Work out the finished part from the listing and answer in its coordinate system (mm). Round coordinates to 2 decimals unless told otherwise and drop trailing zeros. Write each loop counter-clockwise with the first axis right and the second up, starting at its lowest first coordinate (ties: lowest second). Pieces come first, ordered by that corner, then holes. Notation, with made-up numbers: M -40,55 L -35,55 A22 ccw -35,92 Z; hole C 73.25,-22.75 d11. An arc over 180 degrees is marked long. Answer in a Markdown table with one row per item.
```python
from build123d import *

# Parameters (mm, degrees)
SKETCH_1_R          = 10
EXTRUDE_1_DEPTH     = 3
SKETCH_3_R          = 0.75
CUT_EXTRUDE_2_DEPTH = 15.456832295
SKETCH_4_R          = 1.8
CUT_EXTRUDE_3_DEPTH = 15.456832295
CUT_EXTRUDE_6_REACH = 16.457


with BuildPart() as part:
    # 草图1 → 凸台-拉伸1 (new body)
    with BuildSketch(Plane(origin=(0, 0, 0), x_dir=(1, 0, 0), z_dir=(0, 1, 0))):
        with Locations(Location((0, 0, 0), (0, 0, 270))):
            Circle(SKETCH_1_R)
    extrude(amount=EXTRUDE_1_DEPTH)

    # 草图3 → 切除-拉伸2 (cut, through all)
    with BuildSketch(Plane(origin=(0, 3, 0), x_dir=(1, 0, 0), z_dir=(0, 1, 0))):
        with Locations(Location((0, 8, 0), (0, 0, 270))):
            Circle(SKETCH_3_R)
        with Locations(Location((2.736161147, 7.517540966, 0), (0, 0, 270))):
            Circle(SKETCH_3_R)
        with Locations(Location((5.142300877, 6.128355545, 0), (0, 0, 270))):
            Circle(SKETCH_3_R)
        with Locations(Location((6.92820323, 4, 0), (0, 0, 270))):
            Circle(SKETCH_3_R)
        with Locations(Location((7.878462024, 1.389185421, 0), (0, 0, 270))):
            Circle(SKETCH_3_R)
        with Locations(Location((7.878462024, -1.389185421, 0), (0, 0, 270))):
            Circle(SKETCH_3_R)
        with Locations(Location((6.92820323, -4, 0), (0, 0, 270))):
            Circle(SKETCH_3_R)
        with Locations(Location((5.142300877, -6.128355545, 0), (0, 0, 270))):
            Circle(SKETCH_3_R)
        with Locations(Location((2.736161147, -7.517540966, 0), (0, 0, 270))):
            Circle(SKETCH_3_R)
        with Locations(Location((0, -8, 0), (0, 0, 270))):
            Circle(SKETCH_3_R)
        with Locations(Location((-2.736161147, -7.517540966, 0), (0, 0, 270))):
            Circle(SKETCH_3_R)
        with Locations(Location((-5.142300877, -6.128355545, 0), (0, 0, 270))):
            Circle(SKETCH_3_R)
        with Locations(Location((-6.92820323, -4, 0), (0, 0, 270))):
            Circle(SKETCH_3_R)
        with Locations(Location((-7.878462024, -1.389185421, 0), (0, 0, 270))):
            Circle(SKETCH_3_R)
        with Locations(Location((-7.878462024, 1.389185421, 0), (0, 0, 270))):
            Circle(SKETCH_3_R)
        with Locations(Location((-6.92820323, 4, 0), (0, 0, 270))):
            Circle(SKETCH_3_R)
        with Locations(Location((-5.142300877, 6.128355545, 0), (0, 0, 270))):
            Circle(SKETCH_3_R)
        with Locations(Location((-2.736161147, 7.517540966, 0), (0, 0, 270))):
            Circle(SKETCH_3_R)
    extrude(amount=-CUT_EXTRUDE_2_DEPTH, mode=Mode.SUBTRACT)

    # 草图4 → 切除-拉伸3 (cut, through all)
    with BuildSketch(Plane(origin=(0, 3, 0), x_dir=(1, 0, 0), z_dir=(0, 1, 0))):
        with Locations(Location((3, -4, 0), (0, 0, 270))):
            Circle(SKETCH_4_R)
        with Locations(Location((3, 4, 0), (0, 0, 90))):
            Circle(SKETCH_4_R)
    extrude(amount=-CUT_EXTRUDE_3_DEPTH, mode=Mode.SUBTRACT)

    # 草图2 → 切除-拉伸6 (cut, up to next)
    with BuildSketch(Plane(origin=(0, 3, 0), x_dir=(1, 0, 0), z_dir=(0, 1, 0)), mode=Mode.PRIVATE) as cut_extrude_6_sk1:
        with BuildLine():
            Line((1, -1.118033989), (1, 1.118033989))
            ThreePointArc((1, 1.118033989), (-1.5, 0), (1, -1.118033989))
        make_face()
    cut_extrude_6_tool1 = extrude(cut_extrude_6_sk1.sketch, amount=-CUT_EXTRUDE_6_REACH, mode=Mode.PRIVATE) & part.part
    add(cut_extrude_6_tool1.solids().sort_by_distance((-0.148024, 3, 0))[0], mode=Mode.SUBTRACT)


solid = part.part
```
1. The part is cut by section B-B (z = 0). Determine the outline of the cut face in (x, y), plus the area to 3 significant figures.
Calculated:
| item | result |
|---|---|
| outline | M -10,0 L -1.5,0 L -1.5,3 L -10,3 Z; M 1,0 L 10,0 L 10,3 L 1,3 Z |
| area | 52.5 mm² |
2. The part is cut by section C-C (y = 1). Count the separate pieces of the cut face and the enclosed holes in it, plus the area to 3 significant figures.
Calculated:
| item | result |
|---|---|
| separate pieces | 1 |
| enclosed holes | 21 |
| area | 256 mm² |
3. The part is cut by section A-A (x = 0). Determine the outline of the cut face in (y, z).
Calculated:
| item | result |
|---|---|
| outline | M 0,-10 L 3,-10 L 3,-8.75 L 0,-8.75 Z; M 0,-7.25 L 3,-7.25 L 3,-1.5 L 0,-1.5 Z; M 0,1.5 L 3,1.5 L 3,7.25 L 0,7.25 Z; M 0,8.75 L 3,8.75 L 3,10 L 0,10 Z |
4. Consider line 1 along X through (y, z) = (1.5, -8); line 2 along Z through (x, y) = (0.5, 2.2); line 3 along X through (y, z) = (2.05, 2). Determine where each line is inside the solid, lowest interval first. Write a range as from..to.
Calculated:
| item | result |
|---|---|
| line 1 | x = -6..-3.31, -2.16..-0.75, 0.75..2.16, 3.31..6 |
| line 2 | z = -9.99..-8.56, -7.44..-1.41, 1.41..7.44, 8.56..9.99 |
| line 3 | x = -9.8..-8.31, -7.44..7.44, 8.31..9.8 |
5. Determine the mould class of faces 1 (the cylindrical face through (-9.76, 1.48, -2.17)), 2 (the cylindrical face through (2.77, 1.52, 6.77)), 3 (the flat face through (-2, 0, 0)), 4 (the cylindrical face through (-4.917, 1.521, 6.844)) for opening direction X: released by +X, released by -X, zero draft, split by the parting line, or undercut.
Calculated:
| item | result |
|---|---|
| face 1 | split by the parting line |
| face 2 | undercut |
| face 3 | zero draft |
| face 4 | undercut |
6. The part is cut by section D-D (x = 3). Determine the outline of the cut face in (y, z).
Calculated:
| item | result |
|---|---|
| outline | M 0,-9.54 L 3,-9.54 L 3,-8.22 L 0,-8.22 Z; M 0,-6.82 L 3,-6.82 L 3,-5.8 L 0,-5.8 Z; M 0,-2.2 L 3,-2.2 L 3,2.2 L 0,2.2 Z; M 0,5.8 L 3,5.8 L 3,6.82 L 0,6.82 Z; M 0,8.22 L 3,8.22 L 3,9.54 L 0,9.54 Z |
7. Given pin 1 (1.4 mm diameter, centred on x = -5.14, z = -6.13, fed in from +Y); pin 2 (1.5 mm diameter, centred on y = 1.5, z = -1, fed in from -X), each flat-ended and moving along its own axis, determine where each tip first touches the part or whether it passes through.
Calculated:
| item | result |
|---|---|
| pin 1 | passes through |
| pin 2 | stops at x = -10 |
